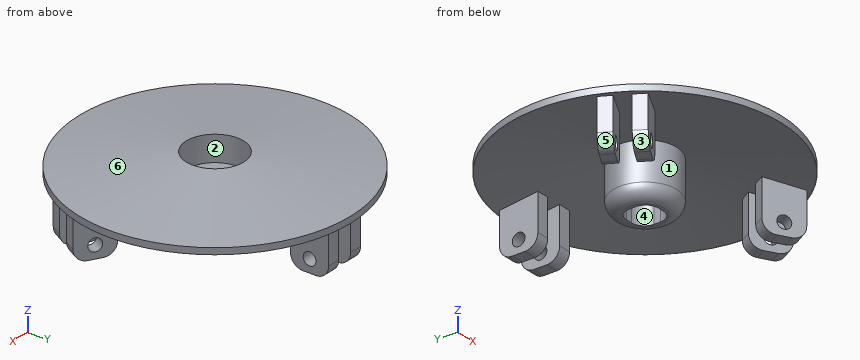
```python
from build123d import *

# Parameters (mm, degrees)
SKETCH1_R                = 22.5
BOSS_EXTRUDE1_DEPTH      = 15
SKETCH4_R                = 25
BOSS_EXTRUDE2_DEPTH      = 30
BOSS_EXTRUDE2_DEPTH_BACK = 10
SKETCH1_3_R              = 22.5
CUT_EXTRUDE1_DEPTH       = 5
SKETCH1_4_R              = 22.5
CUT_EXTRUDE2_DEPTH       = 15
BOSS_EXTRUDE3_START      = -30
SKETCH10_W               = 10
SKETCH10_H               = 30
BOSS_EXTRUDE3_DEPTH      = 39.101444
FILLET1_R                = 10
SKETCH11_R               = 5
CUT_EXTRUDE3_DEPTH       = 32
CIRPATTERN1_COUNT        = 3
FILLET1_OF_CIRPATTERN1_R = 10
FILLET2_R                = 10


with BuildPart() as part:
    # Sketch1 → Boss-Extrude1 (new body)
    with BuildSketch(Plane.XY):
        Circle(SKETCH1_R)
    extrude(amount=BOSS_EXTRUDE1_DEPTH)

    # Sketch3 → Revolve1 (revolve)
    with BuildSketch(Plane(origin=(0, 0, 0), x_dir=(0, 0, -1), z_dir=(1, 0, 0))):
        Polygon((-5, 106.5), (-15, 22.5), (-9.964693814, 22.5), (0, 106.203428035), (0, 106.5), align=None)
    revolve(axis=Axis((0, 0, 15), (0, 0, -1)))

    # Sketch4 → Boss-Extrude2 (add, two sides)
    with BuildSketch(Plane(origin=(0, 0, 0), x_dir=(-1, 0, 0), z_dir=(0, 0, -1))) as boss_extrude2_sk:
        Circle(SKETCH4_R)
        with BuildLine():
            Line((-2.5, 12.5), (2.5, 12.5))
            ThreePointArc((2.5, 12.5), (9.571067812, 9.571067812), (12.5, 2.5))
            Line((12.5, 2.5), (12.5, -2.5))
            ThreePointArc((12.5, -2.5), (9.571067812, -9.571067812), (2.5, -12.5))
            Line((2.5, -12.5), (-2.5, -12.5))
            ThreePointArc((-2.5, -12.5), (-9.571067812, -9.571067812), (-12.5, -2.5))
            Line((-12.5, -2.5), (-12.5, 2.5))
            ThreePointArc((-12.5, 2.5), (-9.571067812, 9.571067812), (-2.5, 12.5))
        make_face(mode=Mode.SUBTRACT)
    extrude(amount=BOSS_EXTRUDE2_DEPTH)
    extrude(boss_extrude2_sk.sketch, amount=-BOSS_EXTRUDE2_DEPTH_BACK)

    # Sketch1<3> → Cut-Extrude1 (cut)
    with BuildSketch(Plane.XY):
        Circle(SKETCH1_3_R)
    extrude(amount=-CUT_EXTRUDE1_DEPTH, mode=Mode.SUBTRACT)

    # Sketch1<4> → Cut-Extrude2 (cut)
    with BuildSketch(Plane.XY):
        Circle(SKETCH1_4_R)
    extrude(amount=CUT_EXTRUDE2_DEPTH, mode=Mode.SUBTRACT)

    # Sketch10 → Boss-Extrude3 (add)
    with BuildSketch(Plane.XY.offset(-5).offset(BOSS_EXTRUDE3_START)):
        with Locations((-11, 86.5)):
            Rectangle(SKETCH10_W, SKETCH10_H)
        with Locations((11, 86.5)):
            Rectangle(SKETCH10_W, SKETCH10_H)
    boss_extrude3 = extrude(amount=BOSS_EXTRUDE3_DEPTH)

    # Fillet1
    fillet1_edges = [part.edges().sort_by_distance(p)[0] for p in [
        (-11, 101.5, -35),
        (-11, 71.5, -35),
        (11, 101.5, -35),
        (11, 71.5, -35),
    ]]
    fillet(fillet1_edges, radius=FILLET1_R)

    # Sketch11 → Cut-Extrude3 (cut)
    with BuildSketch(Plane.ZY.offset(16)):
        with Locations((-25, 86.5)):
            Circle(SKETCH11_R)
    cut_extrude3 = extrude(amount=-CUT_EXTRUDE3_DEPTH, mode=Mode.SUBTRACT)

    # CirPattern1: Boss-Extrude3, Cut-Extrude3 ×3 about axis
    cirpattern1_axis = Axis((0, 0, 0), (0, 0, 1))
    for i in range(1, CIRPATTERN1_COUNT):
        add(boss_extrude3.rotate(cirpattern1_axis, i * 360 / CIRPATTERN1_COUNT))
        add(cut_extrude3.rotate(cirpattern1_axis, i * 360 / CIRPATTERN1_COUNT), mode=Mode.SUBTRACT)

    # Fillet1 of CirPattern1
    fillet1_of_cirpattern1_edges = [part.edges().sort_by_distance(p)[0] for p in [
        (-82.401578484, -60.276279442, -35),
        (-56.420816371, -45.276279442, -35),
        (-93.401578484, -41.223720558, -35),
        (-67.420816371, -26.223720558, -35),
        (93.401578484, -41.223720558, -35),
        (67.420816371, -26.223720558, -35),
        (82.401578484, -60.276279442, -35),
        (56.420816371, -45.276279442, -35),
    ]]
    fillet(fillet1_of_cirpattern1_edges, radius=FILLET1_OF_CIRPATTERN1_R)

    # Fillet2
    fillet2_edges = [part.edges().sort_by_distance(p)[0] for p in [
        (25, 0, -30),
    ]]
    fillet(fillet2_edges, radius=FILLET2_R)


solid = part.part
```
Here's how the part is built. I have some questions about the finished solid (model axes, mm). Face numbers are marked on the shaded views. A direction names the side the tool comes from. Coordinates: 2 decimals unless noted, no trailing zeros. Order: outer loops, then holes, each group sorted by start corner. A loop starts at its lowest first (then second) coordinate and runs counter-clockwise, first axis right, second up.
1) Which directions (+Z, -Z, +X, -X, +Y, -Y) give clear straight access to the entire face, cutting with the end or side of a thin tool? Please do the marked faces 1, 2 and 3.
2) I need wall thicknesses on line 1 (Y direction, x = -9.5, z = -25); line 2 (Y direction, x = -8, z = -25); line 3 (X direction, y = -43, z = -11.5). Which ranges of each line are inside material? Lowest first, please.
3) Imagine slicing it at A-A on z = -9. State how many separate pieces and enclosed holes the cut face has, and give its area (3 significant figures).
4) Imagine slicing it at B-B on x = 0. List the corners of the cut face in (y, z) for me, and give its area (3 significant figures).
5) Will these pins go through, and if not, where does the flat tip stop? pin 1 (12 mm diameter, centred on y = -57.5, z = 0, fed in from -X); pin 2 (1.5 mm diameter, centred on x = -60.5, z = -23.5, fed in from -Y); pin 3 (16 mm diameter, centred on y = 86.5, z = -25, fed in from +X).
6) We'd pull the mould along Y, two halves only. Please class the marked faces 4, 5 and 6: +Y half, -Y half, draft (parallel to the pull), parting line (faces both ways), or undercut.
Response values:
1. face 1: -Z
1. face 2: +Z
1. face 3: -Z, -X, -Y
2. line 1: y = -21.67 to -9.64, 9.64 to 21.67, 71.5 to 81.5, 91.5 to 101.5
2. line 2: y = -22.27 to -10.85, 10.85 to 22.27, 71.5 to 81.5, 91.5 to 101.5
2. line 3: x = -92.38 to -86.48, -62.48 to -57.74, 57.74 to 62.48, 86.48 to 92.38
3. separate pieces: 7
3. enclosed holes: 1
3. area: 3,220 mm2
4. outline: (-106.5, 0) - (-106.2, 0) - (-25, 9.67) - (-25, -20) arc R10 ccw to (-15, -30) - (-12.5, -30) - (-12.5, -5) - (-22.5, -5) - (-22.5, 15) - (-106.5, 5) - close; (12.5, -30) - (15, -30) arc R10 ccw to (25, -20) - (25, 9.67) - (106.2, 0) - (106.5, 0) - (106.5, 5) - (22.5, 15) - (22.5, -5) - (12.5, -5) - close
4. area: 1,500 mm2
5. pin 1: stops at x = -93.22
5. pin 2: stops at y = -53.84
5. pin 3: stops at x = 16
6. face 4: undercut
6. face 5: -Y half
6. face 6: parting line
